Build history of the part. All positions in model axes, mm. Face numbers are marked on the shaded views. A direction names the side the tool comes from. Give positions to 0.01 mm unless a question says otherwise; leave off trailing zeros. Loops run counter-clockwise (first coordinate to the right, second up) from the corner with the lowest first, then second, coordinate; pieces in that order, holes last. Notation, with made-up numbers: M -7.5,-40 L 20.5,-40 A30 cw 20.5,-15 Z; hole C 6,28.25 d11. An arc over 180 degrees is marked long. Answer as a JSON object with one key per item and string values. Group by question number.
1. Slice it at A-A (z = 0). List the corners of the cut face in (x, y).
2. Slice it at D-D (y = 12.5). List the corners of the cut face in (x, z), then the cut area to 3 significant figures.
3. Drill centre lines: line 1 along Z through (x, y) = (-8.5, 4.5); line 2 along Z through (x, y) = (20.5, 3.25); line 3 along Z through (x, y) = (31, 13). Where is each one in solid material? Low to high. Write a range as [from, to].
4. Drop flat-ended pins along their axis: pin 1 Ø2 at (x, y) = (-22.5, 6.5) entering from -Z; pin 2 Ø5 at (x, z) = (29.5, -45.5) entering from +Y; pin 3 Ø2 at (x, z) = (-30.08, -44.85) entering from -Y; pin 4 Ø5 at (y, z) = (3.5, 45.5) entering from -X. Give the stop position or say it passes through.
5. Mould opens along Z. For the marked faces 4, 5 and 6 say: released by +Z, released by -Z, zero draft, split by the parting line, or undercut.
6. 3-axis set-ups, long thin cutter, end or side, ignore diameter. For the marked faces 1, 2 and 3: which of +Z, -Z, +X, -X, +Y, -Y reach the whole face in a straight line?
7. Slice it at B-B (x = 0). List the corners of the cut face in (y, z).
8. Slice it at C-C (y = 5.25). Give the number of separate pieces and of enclosed holes in the cut face, then the cut area to 3 significant figures.
from build123d import *

# Parameters (mm, degrees)
SKETCH1_R           = 57.5
BOSS_EXTRUDE1_DEPTH = 15
SKETCH2_R           = 50
CUT_EXTRUDE1_DEPTH  = 11
SKETCH3_R           = 15
SKETCH3_R_2         = 1.75
CUT_EXTRUDE2_DEPTH  = 15
CUT_EXTRUDE3_START  = -15
CUT_EXTRUDE3_DEPTH  = 15
CHAMFER1_SIZE       = 7
SKETCH5_R           = 3.25
CUT_EXTRUDE4_DEPTH  = 7
SKETCH6_R           = 3.25
CUT_EXTRUDE5_DEPTH  = 55


with BuildPart() as part:
    # Sketch1 → Boss-Extrude1 (new body)
    with BuildSketch(Plane(origin=(0, 0, 0), x_dir=(1, 0, 0), z_dir=(0, 1, 0))):
        with Locations(Location((0, 0, 0), (0, 0, 270))):
            Circle(SKETCH1_R)
    extrude(amount=BOSS_EXTRUDE1_DEPTH)

    # Sketch2 → Cut-Extrude1 (cut)
    with BuildSketch(Plane.XZ):
        with Locations(Location((0, 0, 0), (0, 0, 270))):
            Circle(SKETCH2_R)
    extrude(amount=-CUT_EXTRUDE1_DEPTH, mode=Mode.SUBTRACT)

    # Sketch3 → Cut-Extrude2 (cut)
    with BuildSketch(Plane(origin=(0, 15, 0), x_dir=(1, 0, 0), z_dir=(0, 1, 0))):
        with Locations(Location((0, 0, 0), (0, 0, 270))):
            Circle(SKETCH3_R)
        with Locations(Location((-10.627298131, 52.943937655, 0), (0, 0, 270))):
            Circle(SKETCH3_R_2)
        with Locations(Location((10.442424555, 52.980711296, 0), (0, 0, 270))):
            Circle(SKETCH3_R_2)
        with Locations(Location((29.922382764, 44.951651913, 0), (0, 0, 270))):
            Circle(SKETCH3_R_2)
        with Locations(Location((44.846929444, 30.079111014, 0), (0, 0, 270))):
            Circle(SKETCH3_R_2)
        with Locations(Location((52.943937655, 10.627298131, 0), (0, 0, 270))):
            Circle(SKETCH3_R_2)
        with Locations(Location((52.980711296, -10.442424555, 0), (0, 0, 270))):
            Circle(SKETCH3_R_2)
        with Locations(Location((44.951651913, -29.922382764, 0), (0, 0, 270))):
            Circle(SKETCH3_R_2)
        with Locations(Location((30.079111014, -44.846929444, 0), (0, 0, 270))):
            Circle(SKETCH3_R_2)
        with Locations(Location((10.627298131, -52.943937655, 0), (0, 0, 270))):
            Circle(SKETCH3_R_2)
        with Locations(Location((-10.442424555, -52.980711296, 0), (0, 0, 270))):
            Circle(SKETCH3_R_2)
        with Locations(Location((-29.922382764, -44.951651913, 0), (0, 0, 270))):
            Circle(SKETCH3_R_2)
        with Locations(Location((-44.846929444, -30.079111014, 0), (0, 0, 270))):
            Circle(SKETCH3_R_2)
        with Locations(Location((-52.943937655, -10.627298131, 0), (0, 0, 270))):
            Circle(SKETCH3_R_2)
        with Locations(Location((-52.980711296, 10.442424555, 0), (0, 0, 270))):
            Circle(SKETCH3_R_2)
        with Locations(Location((-44.951651913, 29.922382764, 0), (0, 0, 270))):
            Circle(SKETCH3_R_2)
        with Locations(Location((-30.079111014, 44.846929444, 0), (0, 0, 270))):
            Circle(SKETCH3_R_2)
    extrude(amount=-CUT_EXTRUDE2_DEPTH, mode=Mode.SUBTRACT)

    # Sketch4 → Cut-Extrude3 (cut)
    with BuildSketch(Plane(origin=(0, 15, 0), x_dir=(1, 0, 0), z_dir=(0, 1, 0)).offset(CUT_EXTRUDE3_START)):
        with BuildLine():
            Line((25, 25), (40.658639918, 40.658639918))
            ThreePointArc((40.658639918, 40.658639918), (57.5, 0), (40.658639918, -40.658639918))
            Line((40.658639918, -40.658639918), (25, -25))
            Line((25, -25), (25, 25))
        make_face()
    cut_extrude3 = extrude(amount=CUT_EXTRUDE3_DEPTH, mode=Mode.SUBTRACT)

    # Mirror1: Cut-Extrude3 across plane
    add(cut_extrude3.mirror(Plane(origin=(0, 0, 0), x_dir=(0, 0, 1), z_dir=(1, 0, 0))), mode=Mode.SUBTRACT)

    # Chamfer1
    # the kernel refuses this chamfer: 7 mm, written as the material it adds along each edge
    with BuildSketch(Plane(origin=(0, 11, 0), x_dir=(0.7071067811865475, 0, -0.7071067811865477), z_dir=(0.7071067811865477, 0, 0.7071067811865475))) as chamfer1_piece_1:
        Polygon((50, -CHAMFER1_SIZE), (50 - CHAMFER1_SIZE, 0), (50, 0), align=None)
    revolve(axis=Axis((0, 11, 0), (0, 1, 0)), revolution_arc=90)
    with BuildSketch(Plane(origin=(0, 11, 0), x_dir=(-0.7071067811865476, 0, 0.7071067811865476), z_dir=(-0.7071067811865476, 0, -0.7071067811865476))) as chamfer1_piece_2:
        Polygon((50 - CHAMFER1_SIZE, 0), (50, -CHAMFER1_SIZE), (50, 0), align=None)
    revolve(axis=Axis((0, 11, 0), (0, 1, 0)), revolution_arc=90)
    # the kernel refuses this chamfer: 7 mm, written as the material it takes off along each edge
    with BuildSketch(Plane(origin=(0, 15, 0), x_dir=(0.890570714861766, 0, 0.4548448107108656), z_dir=(0.4548448107108656, 0, -0.890570714861766))) as chamfer1_2_piece_1:
        Polygon((57.5 - CHAMFER1_SIZE, 0), (57.5, CHAMFER1_SIZE), (57.5, 0), align=None)
    revolve(axis=Axis((0, 15, 0), (0, -1, 0)), revolution_arc=125.890100955, mode=Mode.SUBTRACT)
    with BuildSketch(Plane(origin=(0, 15, 0), x_dir=(-0.890570714861766, 0, -0.4548448107108656), z_dir=(-0.4548448107108656, 0, 0.890570714861766))) as chamfer1_2_piece_2:
        Polygon((57.5, CHAMFER1_SIZE), (57.5 - CHAMFER1_SIZE, 0), (57.5, 0), align=None)
    revolve(axis=Axis((0, 15, 0), (0, -1, 0)), revolution_arc=125.890100955, mode=Mode.SUBTRACT)

    # Sketch5 → Cut-Extrude4 (cut)
    with BuildSketch(Plane(origin=(0, 15, 0), x_dir=(1, 0, 0), z_dir=(0, 1, 0))):
        with Locations(Location((-10.627298131, 52.943937655, 0), (0, 0, 270))):
            Circle(SKETCH5_R)
        with Locations(Location((10.442424555, 52.980711296, 0), (0, 0, 270))):
            Circle(SKETCH5_R)
        with Locations(Location((29.922382764, 44.951651913, 0), (0, 0, 270))):
            Circle(SKETCH5_R)
        with Locations((44.846929444, 30.079111014)):
            Circle(SKETCH5_R)
        with Locations((52.943937655, 10.627298131)):
            Circle(SKETCH5_R)
        with Locations((52.980711296, -10.442424555)):
            Circle(SKETCH5_R)
        with Locations((44.951651913, -29.922382764)):
            Circle(SKETCH5_R)
        with Locations(Location((30.079111014, -44.846929444, 0), (0, 0, 270))):
            Circle(SKETCH5_R)
        with Locations(Location((10.627298131, -52.943937655, 0), (0, 0, 270))):
            Circle(SKETCH5_R)
        with Locations(Location((-10.442424555, -52.980711296, 0), (0, 0, 270))):
            Circle(SKETCH5_R)
        with Locations(Location((-29.922382764, -44.951651913, 0), (0, 0, 270))):
            Circle(SKETCH5_R)
        with Locations((-44.846929444, -30.079111014)):
            Circle(SKETCH5_R)
        with Locations((-52.943937655, -10.627298131)):
            Circle(SKETCH5_R)
        with Locations((-52.980711296, 10.442424555)):
            Circle(SKETCH5_R)
        with Locations((-44.951651913, 29.922382764)):
            Circle(SKETCH5_R)
        with Locations(Location((-30.079111014, 44.846929444, 0), (0, 0, 270))):
            Circle(SKETCH5_R)
    extrude(amount=-CUT_EXTRUDE4_DEPTH, mode=Mode.SUBTRACT)

    # Sketch6 → Cut-Extrude5 (cut)
    with BuildSketch(Plane(origin=(0, 15, 0), x_dir=(1, 0, 0), z_dir=(0, 1, 0))):
        with Locations(Location((-10.627298131, 52.943937655, 0), (0, 0, 270))):
            Circle(SKETCH6_R)
        with Locations(Location((10.442424555, 52.980711296, 0), (0, 0, 270))):
            Circle(SKETCH6_R)
        with Locations(Location((-10.442424555, -52.980711296, 0), (0, 0, 270))):
            Circle(SKETCH6_R)
        with Locations(Location((10.627298131, -52.943937655, 0), (0, 0, 270))):
            Circle(SKETCH6_R)
    extrude(amount=-CUT_EXTRUDE5_DEPTH, mode=Mode.SUBTRACT)


solid = part.part
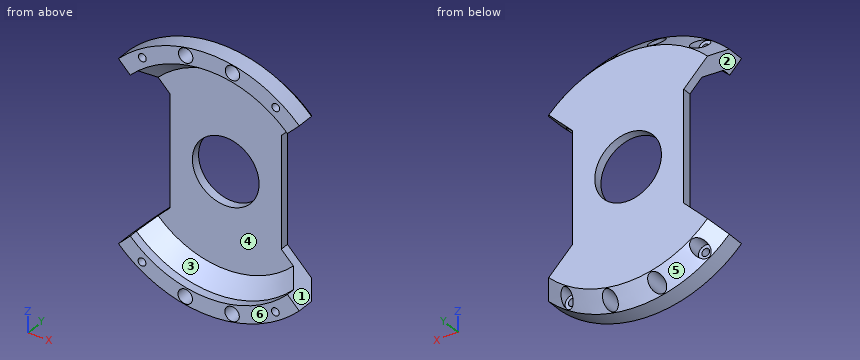
Established:
{
 "1": {"outline": "M -25,11 L -15,11 L -15,15 L -25,15 Z; M 15,11 L 25,11 L 25,15 L 15,15 Z"},
 "2": {"outline": "M -37.48,-37.48 A53 ccw -32.02,-42.24 A3.25 cw -26.93,-45.65 A53 ccw -13.42,-51.27 A3.25 cw -7.41,-52.48 A53 ccw 7.23,-52.5 A3.25 cw 13.24,-51.32 A53 ccw 26.77,-45.74 A3.25 cw 31.87,-42.35 A53 ccw 37.48,-37.48 L 25,-25 L 25,25 L 37.48,37.48 A53 ccw 32.02,42.24 A3.25 cw 26.93,45.65 A53 ccw 13.42,51.27 A3.25 cw 7.41,52.48 A53 ccw -7.23,52.5 A3.25 cw -13.24,51.32 A53 ccw -26.77,45.74 A3.25 cw -31.87,42.35 A53 ccw -37.48,37.48 L -25,25 L -25,-25 Z; hole C 0,0 d30", "area": "4,880 mm^2"},
 "3": {"line 1": "z = [-56.87, -55.4], [-50.49, -48.76], [48.76, 50.38], [55.59, 56.87]", "line 2": "z = [-53.72, -45.6], [45.6, 53.72]", "line 3": "z = [-41.89, -31], [31, 41.73]"},
 "4": {"pin 1": "stops at z = -53.33", "pin 2": "stops at y = 8", "pin 3": "passes through", "pin 4": "stops at x = -38.17"},
 "5": {"face 4": "undercut", "face 5": "released by -Z", "face 6": "zero draft"},
 "6": {"face 1": "+X, +Y, -Y", "face 2": "-X, +Y, -Y", "face 3": "-Y"},
 "7": {"outline": "M 0,-57.5 L 8,-57.5 L 15,-50.5 L 15,-15 L 11,-15 L 11,-43 L 4,-50 L 0,-50 Z; M 0,50 L 4,50 L 11,43 L 11,15 L 15,15 L 15,50.5 L 8,57.5 L 0,57.5 Z"},
 "8": {"separate pieces": "2", "enclosed holes": "8", "area": "1,290 mm^2"}
}
